Design review of the part built by this model. Coordinates are the model's own, in mm. Face numbers are marked on the shaded views. A direction names the side the tool comes from. Coordinates: 2 decimals unless noted, no trailing zeros. Order: outer loops, then holes, each group sorted by start corner. A loop starts at its lowest first (then second) coordinate and runs counter-clockwise, first axis right, second up. Notation, with made-up numbers: M 31.25,-33.75 L 62.25,-33.75 A19 cw 62.25,-14.75 Z; hole C 52.5,37.5 d5. An arc over 180 degrees is marked long. Answer in a Markdown table with one row per item.
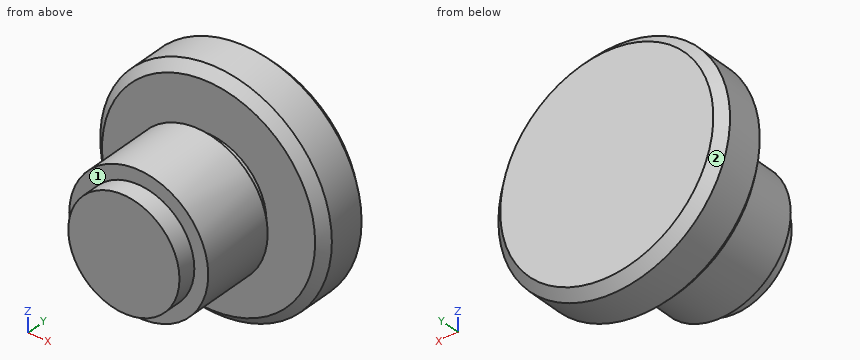
from build123d import *

# Parameters (mm, degrees)
F0_R      = 7.9375
F1_DEPTH  = 3.81
F2_R      = 4.7625
F3_DEPTH  = 6.35
F5_R      = 3.96875
F6_DEPTH  = 0.889
F7_R      = 4.7625
F7_R_2    = 3.96875
F8_DEPTH  = 6.35
F9_R      = 4.7625
F9_R_2    = 3.81
F10_DEPTH = 1.27
F11_SIZE  = 0.635


with BuildPart() as f1:
    # F0 (on Front) → F1 (new body)
    with BuildSketch(Plane.XZ):
        Circle(F0_R)
    extrude(amount=F1_DEPTH)

    # F5 (on face) → F6 (join)
    with BuildSketch(Plane.XZ.offset(3.81)):
        Circle(F5_R)
    extrude(amount=F6_DEPTH)

    # F7 (on face) → F8 (join)
    with BuildSketch(Plane.XZ.offset(4.699)):
        Circle(F7_R)
        Circle(F7_R_2, mode=Mode.SUBTRACT)
        Circle(F7_R_2)
    extrude(amount=F8_DEPTH)

    # F9 (on face) → F10 (cut)
    with BuildSketch(Plane.XZ.offset(11.049)):
        Circle(F9_R)
        Circle(F9_R_2, mode=Mode.SUBTRACT)
    extrude(amount=-F10_DEPTH, mode=Mode.SUBTRACT)

    # F11
    f11_edges = [f1.edges().sort_by_distance(p)[0] for p in [
        (-7.9375, -3.81, 0),
        (-7.9375, 0, 0),
    ]]
    chamfer(f11_edges, length=F11_SIZE)


with BuildPart() as f3:
    # F2 (on face) → F3 (new body)
    with BuildSketch(Plane.XZ.offset(3.81)):
        Circle(F2_R)
    extrude(amount=F3_DEPTH)


solid = f1.part
(1) Add section A-A, the plane x = 0. Give the boundary of the cut face in (y, z) (1 decimal).
Return value:
| item | result |
|---|---|
| outline | M -11,-3.8 L -9.8,-3.8 L -9.8,-4.8 L -4.7,-4.8 L -4.7,-4 L -3.8,-4 L -3.8,-7.3 L -3.2,-7.9 L -0.6,-7.9 L 0,-7.3 L 0,7.3 L -0.6,7.9 L -3.2,7.9 L -3.8,7.3 L -3.8,4 L -4.7,4 L -4.7,4.8 L -9.8,4.8 L -9.8,3.8 L -11,3.8 Z |
(2) Add section C-C, the plane y = -8. Give the boundary of the cut face in (x, z) (1 decimal), and give its area (3 significant figures).
Return value:
| item | result |
|---|---|
| outline | C 0,0 d9.5 |
| area | 71.3 mm2 |
(3) For line 1 along Y through (x, z) = (1.5, 4.25); line 2 along Y through (x, z) = (-1.5, -6); line 3 along X through (y, z) = (-2.75, 0.25), list the stretches that pass through material, from the lowest coordinate up. Write a range as from..to.
Return value:
| item | result |
|---|---|
| line 1 | y = -9.78..-4.7, -3.81..0 |
| line 2 | y = -3.81..0 |
| line 3 | x = -7.93..7.93 |
(4) For the marked faces 1 and 2, list the 3-axis set-ups (+Z, -Z, +X, -X, +Y, -Y) from which the entire face can be reached by the end or side of a thin tool; tool diameter is ignored.
Return value:
| item | result |
|---|---|
| face 1 | -Y |
| face 2 | +Y |
(5) Insertion check: pin 1 Ø5 at (x, z) = (-4, 0.5) entering from +Y; pin 2 Ø1.5 at (x, y) = (-1.5, -6.5) entering from -Z; pin 3 Ø3 at (y, z) = (-2.5, 5.5) entering from +X; pin 4 Ø6 at (x, y) = (1, -9) entering from -Z. Each pin has a flat end and moves straight along its axis. Give the tip position at first contact, or say it passes through.
Return value:
| item | result |
|---|---|
| pin 1 | stops at y = 0 |
| pin 2 | stops at z = -4.7 |
| pin 3 | stops at x = 6.86 |
| pin 4 | stops at z = -4.76 |
(6) Add section B-B, the plane y = -2.75. Give the boundary of the cut face in (x, z) (1 decimal).
Return value:
| item | result |
|---|---|
| outline | C 0,0 d15.9 |
